from build123d import *

# Parameters (mm, degrees)
SKETCH_1_W          = 40
SKETCH_1_H          = 40
SKETCH_1_R          = 3
EXTRUDE_1_DEPTH     = 5
SKETCH_2_W          = 10
SKETCH_2_H          = 40
EXTRUDE_2_DEPTH     = 67.34
SKETCH_3_W          = 10
SKETCH_3_H          = 28
EXTRUDE_3_DEPTH     = 24.5
SKETCH_5_R          = 2
CUT_EXTRUDE_1_DEPTH = 12.25
SKETCH_6_W          = 12
SKETCH_6_H          = 28
CUT_EXTRUDE_2_DEPTH = 2
SKETCH_7_W          = 3
SKETCH_7_H          = 28
CUT_EXTRUDE_3_DEPTH = 25


with BuildPart() as part:
    # 草图1 → 凸台-拉伸1 (new body)
    with BuildSketch(Plane(origin=(0, 0, 0), x_dir=(1, 0, 0), z_dir=(0, 1, 0))):
        Rectangle(SKETCH_1_W, SKETCH_1_H)
        with Locations((-10, -15)):
            Circle(SKETCH_1_R, mode=Mode.SUBTRACT)
        with Locations((10, -15)):
            Circle(SKETCH_1_R, mode=Mode.SUBTRACT)
        with Locations((10, 15)):
            Circle(SKETCH_1_R, mode=Mode.SUBTRACT)
        with Locations((-10, 15)):
            Circle(SKETCH_1_R, mode=Mode.SUBTRACT)
    extrude(amount=EXTRUDE_1_DEPTH)

    # 草图2 → 凸台-拉伸2 (add)
    with BuildSketch(Plane(origin=(0, 5, 0), x_dir=(1, 0, 0), z_dir=(0, 1, 0))):
        Rectangle(SKETCH_2_W, SKETCH_2_H)
    extrude(amount=EXTRUDE_2_DEPTH)

    # 草图3 → 凸台-拉伸3 (add)
    with BuildSketch(Plane.ZY.offset(5)):
        with Locations((0, 58.34)):
            Rectangle(SKETCH_3_W, SKETCH_3_H)
    extrude_3 = extrude(amount=EXTRUDE_3_DEPTH)

    # 草图5 → 切除-拉伸1 (cut, symmetric)
    with BuildSketch(Plane.XY):
        with Locations((-21.41, 68.31)):
            Circle(SKETCH_5_R)
        with Locations((-21.41, 58.49)):
            Circle(SKETCH_5_R)
        with Locations((-21.41, 48.67)):
            Circle(SKETCH_5_R)
    cut_extrude_1 = extrude(amount=CUT_EXTRUDE_1_DEPTH, both=True, mode=Mode.SUBTRACT)

    # 草图6 → 切除-拉伸2 (cut, symmetric)
    with BuildSketch(Plane.XY):
        with Locations((-23.5, 58.34)):
            Rectangle(SKETCH_6_W, SKETCH_6_H)
    cut_extrude_2 = extrude(amount=CUT_EXTRUDE_2_DEPTH, both=True, mode=Mode.SUBTRACT)

    # 镜向1: 凸台-拉伸3, 切除-拉伸1, 切除-拉伸2 across plane
    add(extrude_3.mirror(Plane(origin=(0, 0, 0), x_dir=(0, 0, 1), z_dir=(1, 0, 0))))
    add(cut_extrude_1.mirror(Plane(origin=(0, 0, 0), x_dir=(0, 0, 1), z_dir=(1, 0, 0))), mode=Mode.SUBTRACT)
    add(cut_extrude_2.mirror(Plane(origin=(0, 0, 0), x_dir=(0, 0, 1), z_dir=(1, 0, 0))), mode=Mode.SUBTRACT)

    # 草图7 → 切除-拉伸3 (cut, symmetric)
    with BuildSketch(Plane.XY):
        with Locations((-28, 58.34)):
            Rectangle(SKETCH_7_W, SKETCH_7_H)
    cut_extrude_3 = extrude(amount=CUT_EXTRUDE_3_DEPTH, both=True, mode=Mode.SUBTRACT)

    # 镜向2: 切除-拉伸3 across plane
    add(cut_extrude_3.mirror(Plane(origin=(0, 0, 0), x_dir=(0, 0, 1), z_dir=(1, 0, 0))), mode=Mode.SUBTRACT)


solid = part.part
Design review of the part built by this model. Coordinates are the model's own, in mm. A direction names the side the tool comes from. Round coordinates to 2 decimals unless told otherwise and drop trailing zeros. Write each loop counter-clockwise with the first axis right and the second up, starting at its lowest first coordinate (ties: lowest second). Pieces come first, ordered by that corner, then holes. Notation, with made-up numbers: (-5.75, 85) -> (43.25, 85) arc R25 ccw to (43.25, 119) -> close; hole circle Ø10 at (61.5, 39.5). An arc over 180 degrees is marked (long way). One line per item, written item: value. Start each with the question number.
Q1. Insertion check: P1, Ø12, axis at y = 52, z = -10.5, coming from the +X side; P2, Ø5.5, axis at x = -10, z = -15, coming from the -Y side; P3, Ø5, axis at x = 14.5, z = 8.5, coming from the +Y side; P4, Ø6.5, axis at x = 21.41, y = 68.31, coming from the +Z side. Each pin has a flat end and moves straight along its axis. Give the tip position at first contact, or say it passes through.
Q2. Add section C-C (z = 15). Give the boundary of the cut face in (x, y), then the cut area to 3 significant figures.
Q3. The part is to be moulded in two halves that separate along Y. For faces 6 (the face through (0, 0, 0)), 7 (the face through (-16, 44.34, 0)), 8 (the face through (11.384, 2.465, -12.338)), 9 (the face through (0, 72.34, 0)), say which applies: pulls with the +Y half, pulls with the -Y half, needs draft (parallel to the pull), parting line crosses it, or undercut.
Q4. To check wall thickness, follow probe 1 along Y at (x, z) = (-9, -3); probe 2 along X at (y, z) = (2, 15); probe 3 along X at (y, z) = (68, 3). State the ranges of each line that lie inside material, in increasing order.
Q5. Tool access review of faces 1 (the face through (12, 5, 0)), 2 (the face through (-16, 58, -5)), 3 (the face through (24, 59, -2)), 4 (the face through (16, 58, 5)), 5 (the face through (-24, 59, 2)): name each direction out of +Z, -Z, +X, -X, +Y, -Y from which nothing blocks a thin tool from reaching the whole face with its end or side.
Q6. Add section A-A (x = -21.41). State how many separate pieces and enclosed holes the cut face has, then the cut area to 3 significant figures.
Q7. Add section B-B (x = -10). Give the boundary of the cut face in (y, z), then the cut area to 3 significant figures.
Q8. Add section D-D (z = -3). Give the boundary of the cut face in (x, y), then the cut area to 3 significant figures.
Response:
1. P1: stops at x = 26.5
1. P2: passes through
1. P3: stops at y = 5
1. P4: stops at z = 5
2. outline: (-20, 0) -> (-13, 0) -> (-13, 5) -> (-20, 5) -> close; (-7, 0) -> (7, 0) -> (7, 5) -> (5, 5) -> (5, 72.34) -> (-5, 72.34) -> (-5, 5) -> (-7, 5) -> close; (13, 0) -> (20, 0) -> (20, 5) -> (13, 5) -> close
2. area: 813 mm^2
3. face 6: pulls with the -Y half
3. face 7: undercut
3. face 8: needs draft
3. face 9: pulls with the +Y half
4. probe 1: y = 0 to 5, 44.34 to 72.34
4. probe 2: x = -20 to -13, -7 to 7, 13 to 20
4. probe 3: x = -26.5 to -23.39, -19.43 to 19.43, 23.39 to 26.5
5. face 1: +Z, -Z, +X
5. face 2: -Z, -X, +Y
5. face 3: +X, +Y
5. face 4: +Z, +X, +Y
5. face 5: -X, +Y
6. separate pieces: 8
6. enclosed holes: 0
6. area: 96.0 mm^2
7. outline: (0, -20) -> (5, -20) -> (5, -18) -> (0, -18) -> close; (0, -12) -> (5, -12) -> (5, 12) -> (0, 12) -> close; (0, 18) -> (5, 18) -> (5, 20) -> (0, 20) -> close; (44.34, -5) -> (72.34, -5) -> (72.34, 5) -> (44.34, 5) -> close
7. area: 420 mm^2
8. outline: (-26.5, 44.34) -> (-5, 44.34) -> (-5, 5) -> (-20, 5) -> (-20, 0) -> (20, 0) -> (20, 5) -> (5, 5) -> (5, 44.34) -> (26.5, 44.34) -> (26.5, 72.34) -> (-26.5, 72.34) -> close; hole circle Ø4 at (-21.41, 48.67); hole circle Ø4 at (-21.41, 58.49); hole circle Ø4 at (-21.41, 68.31); hole circle Ø4 at (21.41, 48.67); hole circle Ø4 at (21.41, 58.49); hole circle Ø4 at (21.41, 68.31)
8. area: 2,000 mm^2
